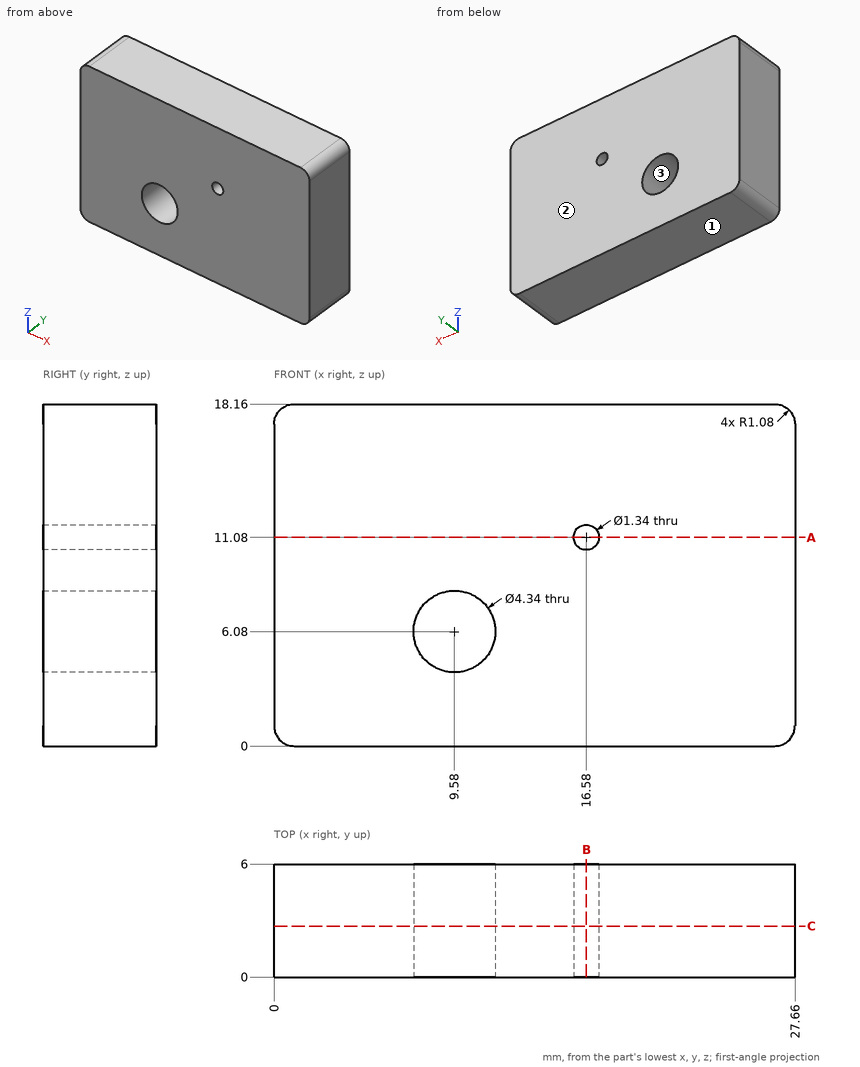
Job drawing, mm, ordinate dimensions from the low corner. One solid piece. Coordinates: 2 decimals unless noted, no trailing zeros. Order: outer loops, then holes, each group sorted by start corner. A loop starts at its lowest first (then second) coordinate and runs counter-clockwise, first axis right, second up. Notation, with made-up numbers: (60, 13) - (117, 13) arc R21 ccw to (117, 20) - close; hole circle Ø5 at (83, 67.5). An arc over 180 degrees is marked (long way). Write each question's results on one line, items separated by ' | '. Start each with the question number.
Item 1: Band-saw the part on C-C on y = 2.7. Write the cut outline in (x, z).
Item 2: Band-saw the part on B-B on x = 16.58. Write the cut outline in (y, z), and give its area (3 significant figures).
Item 3: Band-saw the part on A-A on z = 11.08. Write the cut outline in (x, y), and give its area (3 significant figures).
Item 4: Mould opens along Z. For the marked faces 1, 2 and 3 say: released by +Z, released by -Z, zero draft, split by the parting line, or undercut.
Item 5: Wall check: probe 1 along X at (y, z) = (1.5, 11.08); probe 2 along X at (y, z) = (4.7, 6.08); probe 3 along Z at (x, y) = (17, 0.5). Give the ranges that are in metal, low to high. Write a range as [from, to].
Numbers:
1) outline: (0, 1.08) arc R1.08 ccw to (1.08, 0) - (26.58, 0) arc R1.08 ccw to (27.66, 1.08) - (27.66, 17.08) arc R1.08 ccw to (26.58, 18.16) - (1.08, 18.16) arc R1.08 ccw to (0, 17.08) - close; hole circle Ø4.34 at (9.58, 6.08); hole circle Ø1.34 at (16.58, 11.08)
2) outline: (0, 0) - (6, 0) - (6, 10.41) - (0, 10.41) - close; (0, 11.75) - (6, 11.75) - (6, 18.16) - (0, 18.16) - close | area: 101 mm^2
3) outline: (0, 0) - (15.91, 0) - (15.91, 6) - (0, 6) - close; (17.25, 0) - (27.66, 0) - (27.66, 6) - (17.25, 6) - close | area: 158 mm^2
4) face 1: released by -Z | face 2: zero draft | face 3: undercut
5) probe 1: [0, 15.91], [17.25, 27.66] | probe 2: [0, 7.41], [11.75, 27.66] | probe 3: [0, 10.56], [11.6, 18.16]
